from build123d import *

# Parameters (mm, degrees)
F0_R     = 10.16
F1_DEPTH = 5.842
F2_DEPTH = 5.842
F4_DEPTH = 4.064


# Not quite as in the source:
# - after a boolean that leaves OpenCascade's solid faulty, fix() repairs it
# - ends of sketch curves that miss each other by under 0.0002 mm in the source are joined


with BuildPart() as f1:
    # F0 (on Top) → F1 (new body)
    with BuildSketch(Plane.XY):
        with BuildLine():
            Line((0, 28.9974835998), (0, 38.1))
            ThreePointArc((0, 38.1), (-26.9407683632, 26.9407683632), (-38.1, 0))
            Line((-38.1, 0), (-34.39917941, -16.3800627568))
            ThreePointArc((-34.39917941, -16.3800627568), (-20.3412095138, -32.2156048448), (0, -38.1))
            Line((0, -38.1), (0, 8.6774835998))
            ThreePointArc((0, 8.6774835998), (-10.16, 18.8374835998), (0, 28.9974835998))
        make_face()
        with Locations((-13.8204852119, -19.0573949367)):
            Circle(F0_R, mode=Mode.SUBTRACT)
        with Locations((-20.0619921088, 6.3544651493)):
            Circle(F0_R, mode=Mode.SUBTRACT)
        with BuildLine():
            Line((34.39917941, -16.3800627568), (38.1, 0))
            ThreePointArc((38.1, 0), (26.9407683632, 26.9407683632), (0, 38.1))
            Line((0, 38.1), (0, 28.9974835998))
            ThreePointArc((0, 28.9974835998), (7.1842048969, 26.0216884966), (10.16, 18.8374835998))
            ThreePointArc((10.16, 18.8374835998), (7.1842048969, 11.6532787029), (0, 8.6774835998))
            Line((0, 8.6774835998), (0, -38.1))
            ThreePointArc((0, -38.1), (20.3412095138, -32.2156048448), (34.39917941, -16.3800627568))
        make_face()
        with Locations((13.8204852119, -19.0573949367)):
            Circle(F0_R, mode=Mode.SUBTRACT)
        with Locations((20.0619921088, 6.3544651493)):
            Circle(F0_R, mode=Mode.SUBTRACT)
    extrude(amount=F1_DEPTH)

    # F0 (on Top) → F2 (join)
    with BuildSketch(Plane.XY):
        with BuildLine():
            Line((16.6278202087, -95.0372070074), (34.39917941, -16.3800627568))
            ThreePointArc((34.39917941, -16.3800627568), (20.3412095138, -32.2156048448), (0, -38.1))
            ThreePointArc((0, -38.1), (-20.3412095138, -32.2156048448), (-34.39917941, -16.3800627568))
            Line((-34.39917941, -16.3800627568), (-16.6278202087, -95.0372070074))
            ThreePointArc((-16.6278202087, -95.0372070074), (0, -108.3273427039), (16.6278202087, -95.0372070074))
        make_face()
    extrude(amount=F2_DEPTH)

    # F3 (on face) → F4 (join)
    with BuildSketch(Plane.XY.offset(5.842)):
        with BuildLine():
            Line((5.5590673185, -13.1434644002), (5.6142329033, 0))
            ThreePointArc((5.6142329033, 0), (0, 5.6142329033), (-5.6142329033, 0))
            Line((-5.6142329033, 0), (-5.5590673185, -13.1434644002))
            ThreePointArc((-5.5590673185, -13.1434644002), (-4.1467680929, -15.9517875723), (-3.6604852119, -19.0573949367))
            ThreePointArc((-3.6604852119, -19.0573949367), (-4.1338185981, -22.1223728994), (-5.5097155096, -24.9017688941))
            Line((-5.5097155096, -24.9017688941), (-5.2310197557, -91.3023650429))
            ThreePointArc((-5.2310197557, -91.3023650429), (-0.0109778096, -86.0493551595), (5.2310658314, -91.280409472))
            Line((5.2310658314, -91.280409472), (5.5097155096, -24.9017688941))
            ThreePointArc((5.5097155096, -24.9017688941), (3.660574702, -19.014751887), (5.5590673185, -13.1434644002))
        make_face()
        with BuildLine():
            ThreePointArc((5.2310197557, -91.3023650429), (5.2310543125, -91.2913872816), (5.2310658314, -91.280409472))
            ThreePointArc((5.2310658314, -91.280409472), (-0.0109778096, -86.0493551595), (-5.2310197557, -91.3023650429))
            ThreePointArc((-5.2310197557, -91.3023650429), (0, -96.5114753034), (5.2310197557, -91.3023650429))
        make_face()
    extrude(amount=F4_DEPTH)

    add(f1.part.fix(), mode=Mode.REPLACE)


solid = f1.part
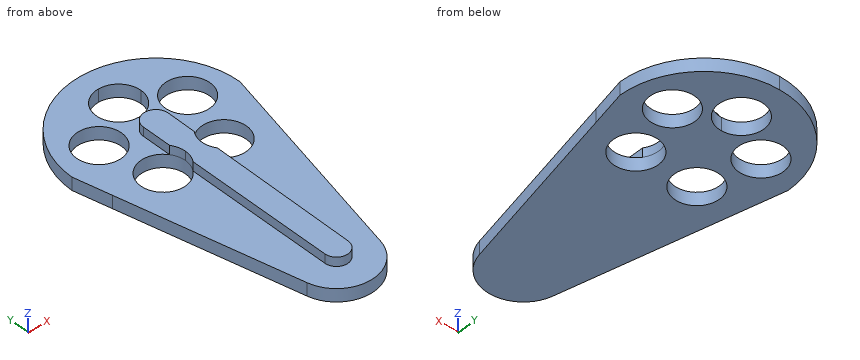
Geometry: final body of the model. Coordinates: model frame, mm. Coordinates: 2 decimals unless noted, no trailing zeros. Write each loop counter-clockwise with the first axis right and the second up, starting at its lowest first coordinate (ties: lowest second). Pieces come first, ordered by that corner, then holes. Notation, with made-up numbers: (-12, 76.25) - (47, 76.25) arc R18 cw to (47, 90.25) - close; hole circle Ø9 at (-28, -39). An arc over 180 degrees is marked (long way). Return JSON: item names as keys, results as strings.
Item 1: Section query A-A (y = -93). Output: boundary loops of the cut face in (x, z), and give its area (3 significant figures).
Completed:
{"outline": "(-17.09, 0) - (17.09, 0) - (17.09, 5.84) - (4.94, 5.84) - (4.94, 9.91) - (-4.94, 9.91) - (-4.94, 5.84) - (-17.09, 5.84) - close", "area": "240 mm2"}
Item 2: Pin query (flat end, axial travel): pin 1 Ø4 at (x, z) = (11, 5.5) entering from +Y; pin 2 Ø2 at (x, y) = (-13, -67) entering from +Z; pin 3 Ø2 at (x, z) = (3.5, 7) entering from -Y. Return the tip coordinate at first contact, or that it passes through.
Completed:
{"pin 1": "stops at y = 37.02", "pin 2": "stops at z = 5.84", "pin 3": "stops at y = -95.88"}
Item 3: Section query C-C (y = -67). Output: boundary loops of the cut face in (x, z).
Completed:
{"outline": "(-22.96, 0) - (22.96, 0) - (22.96, 5.84) - (5.33, 5.84) - (5.33, 9.91) - (-5.33, 9.91) - (-5.33, 5.84) - (-22.96, 5.84) - close"}
Item 4: Line query: L1, parallel to X at y = 12, z = 3.5; L2, parallel to Z at x = 10.5, y = -53.5; L3, parallel to X at y = -23, z = 3.5. Output: solid intervals per line, ascending.
Completed:
{"L1": "x = -36.16 to -28.51, -11.61 to -7.51, 7.51 to 11.61, 28.51 to 36.16", "L2": "z = 0 to 5.84", "L3": "x = -32.9 to -23.18, -4.46 to 4.46, 23.18 to 32.9"}
